```python
from build123d import *

# Parameters (mm, degrees)
F4_DEPTH  = 25.4
F8_DEPTH  = 25.401
F10_DEPTH = 25.401
F11_DEPTH = 25.4


with BuildPart() as f4:
    # F3 (on Top) → F4 (new body)
    with BuildSketch(Plane.XY):
        Polygon((38.1, 29.329394), (-38.1, 29.329394), (-44.45, 18.330871), (-6.35, -47.660265), (6.35, -47.660265), (44.45, 18.330871), align=None)
    extrude(amount=F4_DEPTH)

    # F7 (on Top) → F8 (cut, through all)
    with BuildSketch(Plane.XY):
        Polygon((-3.175, 9.165436), (-9.525, -1.833087), (-6.35, -7.332348), (6.35, -7.332348), (9.525, -1.833087), (3.175, 9.165436), align=None)
    extrude(amount=F8_DEPTH, mode=Mode.SUBTRACT)

    # F9 (on Top) → F10 (cut, through all)
    with BuildSketch(Plane.XY):
        Polygon((39.290625, 17.185192), (34.528125, 25.434084), (30.95625, 21.538773), (34.13125, 16.039512), align=None)
        Polygon((28.971875, 14.893833), (27.384375, 17.643463), (23.8125, 13.748153), align=None)
        Polygon((-30.95625, 21.538773), (-34.528125, 25.434084), (-39.290625, 17.185192), (-34.13125, 16.039512), align=None)
        Polygon((-27.384375, 17.643463), (-28.971875, 14.893833), (-23.8125, 13.748153), align=None)
        Polygon((0, -27.496307), (-1.5875, -32.537296), (1.5875, -32.537296), align=None)
        Polygon((3.175, -37.578286), (-3.175, -37.578286), (-4.7625, -42.619275), (4.7625, -42.619275), align=None)
        Polygon((-7.1625, 24.026792), (-7.975, 25.434084), (-7.1625, 26.841375), (-0.635, 26.841375), (-0.635, 27.476375), (-7.529117, 27.476375), (-8.708235, 25.434084), (-7.529117, 23.391792), (7.529117, 23.391792), (8.708235, 25.434084), (7.529117, 27.476375), (0, 27.476375), (0, 26.841375), (7.1625, 26.841375), (7.975, 25.434084), (7.1625, 24.026792), align=None)
        Polygon((-7.1625, 26.841375), (-7.975, 25.434084), (-7.1625, 24.026792), (7.1625, 24.026792), (7.975, 25.434084), (7.1625, 26.841375), (0, 26.841375), (0, 27.476375), (-0.635, 27.476375), (-0.635, 26.841375), align=None)
    extrude(amount=F10_DEPTH, mode=Mode.SUBTRACT)

    # F9 (on Top) → F11 (join)
    with BuildSketch(Plane.XY):
        Polygon((-7.1625, 26.841375), (-7.975, 25.434084), (-7.1625, 24.026792), (7.1625, 24.026792), (7.975, 25.434084), (7.1625, 26.841375), (0, 26.841375), (0, 27.476375), (-0.635, 27.476375), (-0.635, 26.841375), align=None)
    extrude(amount=F11_DEPTH)


solid = f4.part
```
CAD build for the part. Positions are in the model's coordinates, mm. A direction names the side the tool comes from. Round coordinates to 2 decimals unless told otherwise and drop trailing zeros. Loops run counter-clockwise (first coordinate to the right, second up) from the corner with the lowest first, then second, coordinate; pieces in that order, holes last. Notation, with made-up numbers: (75.25, 55) - (99.25, 55) arc R20 ccw to (99.25, 67) - close; hole circle Ø4 at (-1.75, 10.25). An arc over 180 degrees is marked (long way). Return JSON: item names as keys, results as strings. Group by question number.
Q1. Two-plate mould, pull along X, no slides. Class faces 3 (the face through (7.915, -4.621, 12.522)), 4 (the face through (41.32, 23.75, 12.52)), 5 (the face through (0, -47.66, 13)): +X half, -X half, draft (parallel to the pull), parting line (faces both ways), or undercut.
Q2. Band-saw the part on C-C on z = 11.5. Give the number of separate pieces and of enclosed holes in the cut face, plus the area to 3 significant figures.
Q3. Band-saw the part on B-B on x = -32. Give the cut face in (y, z), plus the area to 3 significant figures.
Q4. Tool access for faces 1 (the face through (-8.13, 24.43, 12.52)), 2 (the face through (-11, 0, 25.4)): list every direction of +Z, -Z, +X, -X, +Y, -Y with a clear straight run to the whole face (end or side of a thin tool).
Q5. Drill centre lines: line 1 along X through (y, z) = (18, 8); line 2 along Y through (x, z) = (-6.5, 4); line 3 along Y through (x, z) = (36.5, 11). Where is each one in solid material? Low to high. Write a range as [from, to].
Q6. Band-saw the part on A-A on y = -30. Give the cut face in (x, z), plus the area to 3 significant figures.
Q7. Flat gauge pins, fed straight in: pin 1 Ø3 at (x, z) = (-22.5, 19.5) entering from -Y; pin 2 Ø6 at (x, y) = (-19, -1) entering from -Z; pin 3 Ø4 at (y, z) = (-22, 20) entering from -X. Where does each tip first touch, or does it go through?
Q8. Band-saw the part on D-D on y = -20.5. Give the cut face in (x, z).
Solutions:
{
 "1": {"face 3": "undercut", "face 4": "+X half", "face 5": "draft"},
 "2": {"separate pieces": "1", "enclosed holes": "8", "area": "3,870 mm^2"},
 "3": {"outline": "(-3.23, 0) - (19.73, 0) - (19.73, 25.4) - (-3.23, 25.4) - close; (22.68, 0) - (29.33, 0) - (29.33, 25.4) - (22.68, 25.4) - close", "area": "752 mm^2"},
 "4": {"face 1": "+Z, -Z", "face 2": "+Z, +X, -X, +Y, -Y"},
 "5": {"line 1": "x = [-44.26, -38.82], [-33, 33], [38.82, 44.26]", "line 2": "y = [-47.4, -7.07], [3.41, 23.39], [24.03, 26.84], [27.48, 29.33]", "line 3": "y = [4.56, 16.57], [22.02, 29.33]"},
 "6": {"outline": "(-16.55, 0) - (-0.79, 0) - (-0.79, 25.4) - (-16.55, 25.4) - close; (0.79, 0) - (16.55, 0) - (16.55, 25.4) - (0.79, 25.4) - close", "area": "800 mm^2"},
 "7": {"pin 1": "stops at y = -22.29", "pin 2": "stops at z = 0", "pin 3": "stops at x = -22.32"},
 "8": {"outline": "(-22.03, 0) - (22.03, 0) - (22.03, 25.4) - (-22.03, 25.4) - close"}
}
